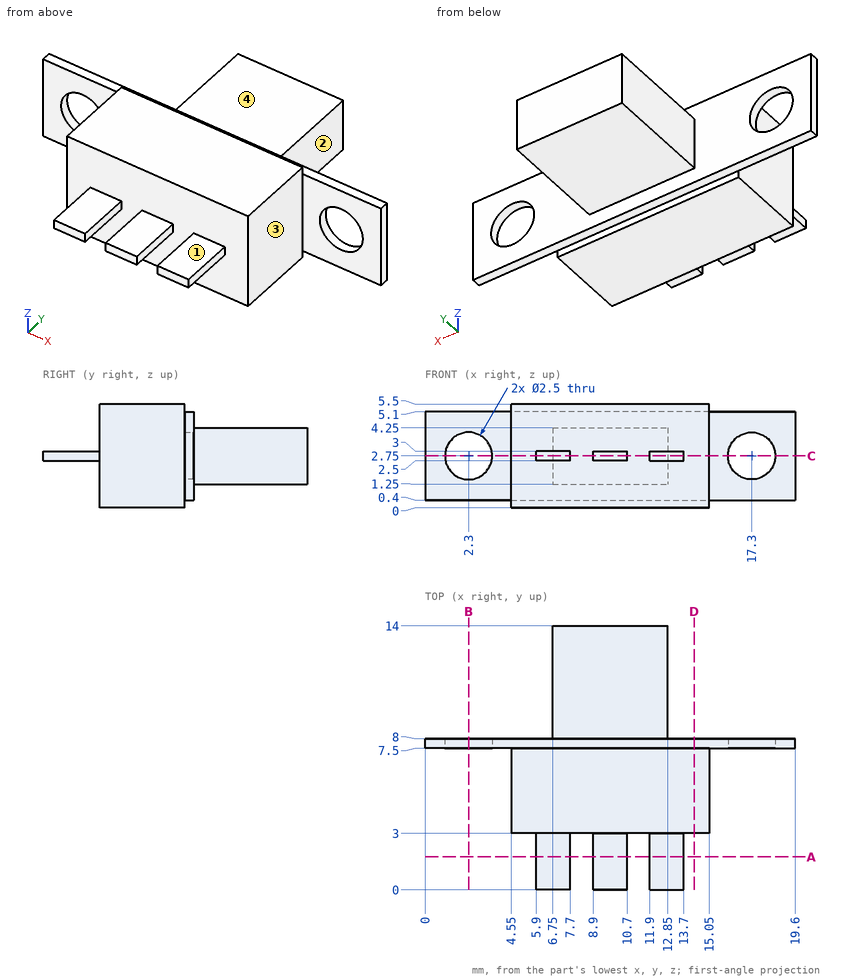
The drawing under review shows one solid part. Ordinate dimensions are in mm from its lowest x, y, z. A direction names the side the tool comes from. Coordinates: 2 decimals unless noted, no trailing zeros. Write each loop counter-clockwise with the first axis right and the second up, starting at its lowest first coordinate (ties: lowest second). Pieces come first, ordered by that corner, then holes. Notation, with made-up numbers: M 14,86.25 L 22,86.25 A23 cw 22,99.25 Z; hole C 46,84 d10. An arc over 180 degrees is marked long. Answer as a JSON object with one key per item and string values.
Item 1: Add section C-C, the plane z = 2.75. State how many separate pieces and enclosed holes the cut face has, and give its area (3 significant figures).
Outcome:
{"separate pieces": "3", "enclosed holes": "0", "area": "107 mm²"}
Item 2: Add section D-D, the plane x = 14.25. Give the boundary of the cut face in (y, z).
Outcome:
{"outline": "M 3,0 L 7.5,0 L 7.5,0.4 L 8,0.4 L 8,5.1 L 7.5,5.1 L 7.5,5.5 L 3,5.5 Z"}
Item 3: Wall thickness on probe 1 along X at (y, z) = (7.7, 2.75); probe 2 along Y at (x, z) = (7.75, 4.1); probe 3 along X at (y, z) = (10.75, 3.7): over which ranges is each line inside the solid? List them lowest first.
Outcome:
{"probe 1": "0 to 1.05, 3.55 to 16.05, 18.55 to 19.6", "probe 2": "3 to 14", "probe 3": "6.75 to 12.85"}
Item 4: Add section B-B, the plane x = 2.3. Give the boundary of the cut face in (y, z), and give its area (3 significant figures).
Outcome:
{"outline": "M 7.5,0.4 L 8,0.4 L 8,1.5 L 7.5,1.5 Z; M 7.5,4 L 8,4 L 8,5.1 L 7.5,5.1 Z", "area": "1.10 mm²"}
Item 5: Insertion check: pin 1 Ø0.9 at (x, y) = (9.5, 1.5) entering from +Z; pin 2 Ø5 at (x, y) = (8.5, 9.5) entering from -Z; pin 3 Ø1 at (x, z) = (3.5, 4.5) entering from +Y; pin 4 Ø1 at (y, z) = (4.5, 4) entering from +X. Each pin has a flat end and moves straight along its axis. Give the tip position at first contact, or say it passes through.
Outcome:
{"pin 1": "z = 3", "pin 2": "z = 0", "pin 3": "y = 8", "pin 4": "x = 15.05"}
Item 6: Add section A-A, the plane y = 1.75. Give the boundary of the cut face in (x, z).
Outcome:
{"outline": "M 5.9,2.5 L 7.7,2.5 L 7.7,3 L 5.9,3 Z; M 8.9,2.5 L 10.7,2.5 L 10.7,3 L 8.9,3 Z; M 11.9,2.5 L 13.7,2.5 L 13.7,3 L 11.9,3 Z"}
Item 7: Machinability: for the marked faces 1, 2, 3 and 4, which of the approach directions +Z, -Z, +X, -X, +Y, -Y give a long, thin tool a straight path to every point of the face, cutting with its end or side? Answer none if there is none.
Outcome:
{"face 1": "+Z, +X, -X, -Y", "face 2": "+Z, -Z, +X, +Y", "face 3": "+Z, -Z, +X, -Y", "face 4": "+Z, +X, -X, +Y"}
